Geometry check sheet. Reference: the model listing, model coordinates, mm. Face numbers are marked on the shaded views. Round coordinates to 2 decimals unless told otherwise and drop trailing zeros. Write each loop counter-clockwise with the first axis right and the second up, starting at its lowest first coordinate (ties: lowest second). Pieces come first, ordered by that corner, then holes. Notation, with made-up numbers: (15.5, 81.25) -> (73.5, 81.25) arc R6 cw to (73.5, 85.25) -> close; hole circle Ø4 at (85.25, -11.5). An arc over 180 degrees is marked (long way). Use a Markdown table: item, result.
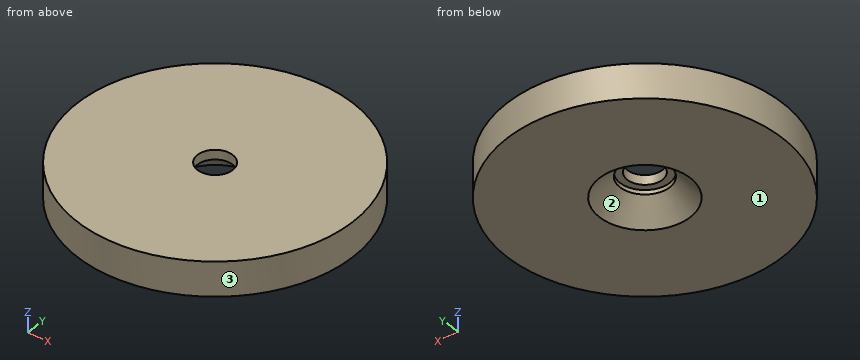
```python
from build123d import *

# Parameters (mm, degrees)
SKETCH1_R           = 9.144
BOSS_EXTRUDE1_DEPTH = 2.286


with BuildPart() as part:
    # Sketch1 → Boss-Extrude1 (new body)
    with BuildSketch(Plane.XY):
        Circle(SKETCH1_R)
    extrude(amount=BOSS_EXTRUDE1_DEPTH)

    # Sketch7 → CBORE for #1 Binding Head Machine Screw2 (revolve, cut)
    with BuildSketch(Plane.YZ):
        Polygon((0, 0), (0, 2.286), (1.1684, 2.286), (1.1684, 1.651), (1.651, 1.651), (1.651, 1.36525), (3.01625, 0), align=None)
    revolve(axis=Axis((0, 0, -6.35), (0, 0, 1)), mode=Mode.SUBTRACT)


solid = part.part
```
(1) Thickness scan on line 1 (Y direction, x = 0, z = 2); line 2 (X direction, y = -1.5, z = 0.8); line 3 (Y direction, x = 0.75, z = 0.85). Record the ranges inside material, lowest first.
A:
| item | result |
|---|---|
| line 1 | y = -9.14 to -1.17, 1.17 to 9.14 |
| line 2 | x = -9.02 to -1.63, 1.63 to 9.02 |
| line 3 | y = -9.11 to -2.03, 2.03 to 9.11 |
(2) Gauge pin test, flat end, axial feed: pin 1 Ø1 at (x, y) = (0, 0) entering from -Z. Record the tip position at first contact, or that the pin passes through.
A:
| item | result |
|---|---|
| pin 1 | passes through |
(3) Section check D-D on y = -8. Record the cut outline in (x, z).
A:
| item | result |
|---|---|
| outline | (-4.43, 0) -> (4.43, 0) -> (4.43, 2.29) -> (-4.43, 2.29) -> close |
(4) Section check A-A on x = 0. Record the cut outline in (y, z).
A:
| item | result |
|---|---|
| outline | (-9.14, 0) -> (-3.02, 0) -> (-1.65, 1.37) -> (-1.65, 1.65) -> (-1.17, 1.65) -> (-1.17, 2.29) -> (-9.14, 2.29) -> close; (1.17, 1.65) -> (1.65, 1.65) -> (1.65, 1.37) -> (3.02, 0) -> (9.14, 0) -> (9.14, 2.29) -> (1.17, 2.29) -> close |
(5) Section check C-C on z = 0.95. Record the cut outline in (x, y), plus the area to 3 significant figures.
A:
| item | result |
|---|---|
| outline | circle Ø18.29 at (0, 0); hole circle Ø4.13 at (0, 0) |
| area | 249 mm2 |
(6) Release check for a two-part mould opening along Y. For the marked faces 1, 2 and 3 record: +Y half, -Y half, draft (parallel to the pull), parting line (faces both ways), or undercut.
A:
| item | result |
|---|---|
| face 1 | draft |
| face 2 | undercut |
| face 3 | parting line |
